Job drawing, mm, ordinate dimensions from the low corner. One solid piece. A direction names the side the tool comes from. Give positions to 0.01 mm unless a question says otherwise; leave off trailing zeros. Write each loop counter-clockwise with the first axis right and the second up, starting at its lowest first coordinate (ties: lowest second). Pieces come first, ordered by that corner, then holes. Notation, with made-up numbers: (85, 61.5) - (103, 61.5) arc R32 ccw to (103, 91.5) - close; hole circle Ø5 at (82, 59.5). An arc over 180 degrees is marked (long way). Answer as a JSON object with one key per item and string values.
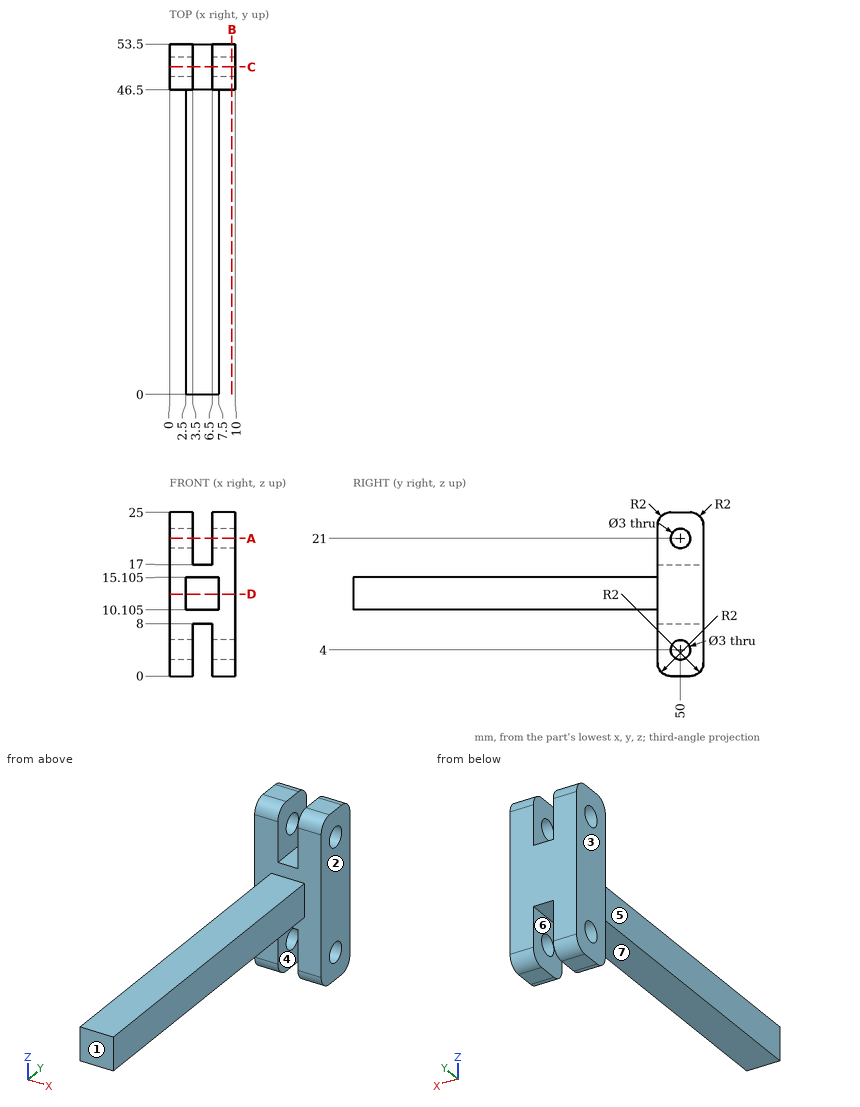
Item 1: Cut at B-B (x = 9.5). Give the cut face in (y, z), and give its area (3 significant figures).
Entries:
{"outline": "(46.5, 2) arc R2 ccw to (48.5, 0) - (51.5, 0) arc R2 ccw to (53.5, 2) - (53.5, 23) arc R2 ccw to (51.5, 25) - (48.5, 25) arc R2 ccw to (46.5, 23) - close; hole circle Ø3 at (50, 4); hole circle Ø3 at (50, 21)", "area": "157 mm2"}
Item 2: Which spindle directions (+Z, -Z, +X, -X, +Y, -Y) get a long thin tool onto all of the face, cutting with end or side? Do the marked faces 5, 6 and 7. Say none if no direction does.
Entries:
{"face 5": "+Z, -Z, -X, -Y", "face 6": "-Z, +Y, -Y", "face 7": "-Z, +X, -X, -Y"}
Item 3: Probe line 1 (Z direction, x = 0.5, y = 50); line 2 (Y direction, x = 8.75, z = 4); line 3 (X direction, y = 50, z = 19). List the from-to ranges inside material, lowest first. Write a range as from..to.
Entries:
{"line 1": "0..2.5, 5.5..19.5, 22.5..25", "line 2": "46.5..48.5, 51.5..53.5", "line 3": "0..3.5, 6.5..10"}
Item 4: Cut at A-A (z = 21). Give the cut face in (x, y), and give its area (3 significant figures).
Entries:
{"outline": "(0, 46.5) - (3.5, 46.5) - (3.5, 48.5) - (0, 48.5) - close; (0, 51.5) - (3.5, 51.5) - (3.5, 53.5) - (0, 53.5) - close; (6.5, 46.5) - (10, 46.5) - (10, 48.5) - (6.5, 48.5) - close; (6.5, 51.5) - (10, 51.5) - (10, 53.5) - (6.5, 53.5) - close", "area": "28.0 mm2"}
Item 5: Mould opens along X. For the marked faces 1, 2, 3 and 4 say: +X half, -X half, draft (parallel to the pull), parting line (faces both ways), or undercut.
Entries:
{"face 1": "draft", "face 2": "+X half", "face 3": "-X half", "face 4": "undercut"}
Item 6: Cut at C-C (y = 50). Give the cut face in (x, z).
Entries:
{"outline": "(0, 0) - (3.5, 0) - (3.5, 2.5) - (0, 2.5) - close; (0, 5.5) - (3.5, 5.5) - (3.5, 8) - (6.5, 8) - (6.5, 5.5) - (10, 5.5) - (10, 19.5) - (6.5, 19.5) - (6.5, 17) - (3.5, 17) - (3.5, 19.5) - (0, 19.5) - close; (0, 22.5) - (3.5, 22.5) - (3.5, 25) - (0, 25) - close; (6.5, 0) - (10, 0) - (10, 2.5) - (6.5, 2.5) - close; (6.5, 22.5) - (10, 22.5) - (10, 25) - (6.5, 25) - close"}
Item 7: Flat gauge pins, fed straight in: P1, Ø4, axis at x = 6, y = 15, coming from the -Z side (3 decimals); P2, Ø1, axis at x = 7, y = 34, coming from the +Z side (3 decimals); P3, Ø1.5, axis at y = 20, z = 13.5, coming from the +X side; P4, Ø2.5, axis at y = 50, z = 4, coming from the +X side. Where does each tip first touch, or does it go through?
Entries:
{"P1": "z = 10.105", "P2": "z = 15.105", "P3": "x = 7.5", "P4": "through"}
Item 8: Cut at D-D (z = 12.5). Give the cut face in (x, y).
Entries:
{"outline": "(0, 46.5) - (2.5, 46.5) - (2.5, 0) - (7.5, 0) - (7.5, 46.5) - (10, 46.5) - (10, 53.5) - (0, 53.5) - close"}
